Part model, mm, in its own coordinate system. Round coordinates to 2 decimals unless told otherwise and drop trailing zeros. Write each loop counter-clockwise with the first axis right and the second up, starting at its lowest first coordinate (ties: lowest second). Pieces come first, ordered by that corner, then holes. Notation, with made-up numbers: M 37.25,73 L 93.25,73 A24 ccw 93.25,96 Z; hole C -25.75,15.25 d9. An arc over 180 degrees is marked long. Use one line per item in the form item = value. Start each with the question number.
Item 1: Cut at C-C, the plane z = 8.25. Give the cut face in (x, y), then the cut area to 3 significant figures.
Item 2: Probe L1, parallel to Z at x = 0, y = -0.4; L2, parallel to X at y = 1.1, z = 9.5; L3, parallel to Z at x = 2.25, y = -1. List the from-to ranges inside material, lowest first.
Item 3: Flat gauge pins, fed straight in: pin 1 Ø3.5 at (x, z) = (0, 9.1) entering from +Y; pin 2 Ø1.5 at (y, z) = (-1, 10.5) entering from +X. Where does each tip first touch, or does it go through?
Item 4: Mould opens along X. For faces 1 (the face through (-5.361, 0.021, 14.245)), 2 (the face through (0.596, 0.021, 6.415)), 3 (the face through (7.5, 0, 4)) say: +X half, -X half, draft (parallel to the pull), parting line (faces both ways), or undercut.
Item 5: Cut at B-B, the plane x = -0.5. Give the cut face in (y, z), then the cut area to 3 significant figures.
Item 6: Cut at D-D, the plane z = 12.25. Give the cut face in (x, y), then the cut area to 3 significant figures.
from build123d import *

# Parameters (mm, degrees)
F0_W     = 15
F0_H     = 3
F1_DEPTH = 16.5
F2_R     = 2.75
F3_DEPTH = 25
F4_R     = 7.49999


# Not quite as in the source:
# - a fillet or chamfer is up to 0.001 mm smaller than in the source, because OpenCascade refuses the exact size


with BuildPart() as f1:
    # F0 (on Top) → F1 (new body)
    with BuildSketch(Plane.XY):
        Rectangle(F0_W, F0_H)
    extrude(amount=F1_DEPTH)

    # F2 (on face) → F3 (cut)
    with BuildSketch(Plane(origin=(0, 1.5, 0), x_dir=(-1, 0, 0), z_dir=(0, 1, 0))):
        with Locations((0, 9.1)):
            Circle(F2_R)
    extrude(amount=-F3_DEPTH, mode=Mode.SUBTRACT)

    # F4 (radius 7.5 in the source; OpenCascade refuses exactly that, so slightly less here)
    f4_edges = [f1.edges().sort_by_distance(p)[0] for p in [
        (-7.5, 0, 16.5),
        (7.5, 0, 16.5),
    ]]
    fillet(f4_edges, radius=F4_R)


solid = f1.part
Model answer:
q1.outline = M -7.5,-1.5 L -2.62,-1.5 L -2.62,1.5 L -7.5,1.5 Z; M 2.62,-1.5 L 7.5,-1.5 L 7.5,1.5 L 2.62,1.5 Z
q1.area = 29.3 mm²
q2.L1 = 0 to 6.35, 11.85 to 16.5
q2.L2 = -7.48 to -2.72, 2.72 to 7.48
q2.L3 = 0 to 7.52, 10.68 to 16.15
q3.pin_1 = through
q3.pin_2 = 7.46
q4.face_1 = -X half
q4.face_2 = undercut
q4.face_3 = +X half
q5.outline = M -1.5,0 L 1.5,0 L 1.5,6.4 L -1.5,6.4 Z; M -1.5,11.8 L 1.5,11.8 L 1.5,16.48 L -1.5,16.48 Z
q5.area = 33.2 mm²
q6.outline = M -6.76,-1.5 L 6.76,-1.5 L 6.76,1.5 L -6.76,1.5 Z
q6.area = 40.6 mm²
